```python
from build123d import *

# Parameters (mm, degrees)
CROQUIS1_R              = 13
CROQUIS1_R_2            = 5
SALIENTE_EXTRUIR1_DEPTH = 8
CHAFL_N1_SIZE           = 0.3
CROQUIS2_W              = 1
CROQUIS2_H              = 0.2


with BuildPart() as part:
    # Croquis1 → Saliente-Extruir1 (new body)
    with BuildSketch(Plane.XY):
        Circle(CROQUIS1_R)
        Circle(CROQUIS1_R_2, mode=Mode.SUBTRACT)
    extrude(amount=SALIENTE_EXTRUIR1_DEPTH)

    # Chaflán1
    chafl_n1_edges = [part.edges().sort_by_distance(p)[0] for p in [
        (-13, 0, 0),
        (-13, 0, 8),
        (-5, 0, 0),
        (-5, 0, 8),
    ]]
    chamfer(chafl_n1_edges, length=CHAFL_N1_SIZE)

    # Croquis2 → Cortar-Revolución1 (revolve, cut)
    with BuildSketch(Plane(origin=(0, 0, 0), x_dir=(0, 0, -1), z_dir=(1, 0, 0))):
        Polygon((-8.85, 11.267505128), (-7.85, 11.142505128), (-7.85, 10.892505128), (-8.85, 10.767505128), align=None)
        Polygon((0.85, 10.767505128), (0.85, 11.267505128), (-0.15, 11.142505128), (-0.15, 10.892505128), align=None)
        with Locations((-8.35, 7.665073065)):
            Rectangle(CROQUIS2_W, CROQUIS2_H)
        with Locations((0.35, 7.665073065)):
            Rectangle(CROQUIS2_W, CROQUIS2_H)
    revolve(axis=Axis((0, 0, 12.411349243), (0, 0, -1)), mode=Mode.SUBTRACT)


solid = part.part
```
Geometry: final body of the model. Coordinates: model frame, mm. Give positions to 0.01 mm unless a question says otherwise; leave off trailing zeros. Order: outer loops, then holes, each group sorted by start corner. A loop starts at its lowest first (then second) coordinate and runs counter-clockwise, first axis right, second up. Notation, with made-up numbers: M 22.25,-7.75 L 57.25,-7.75 A13 cw 57.25,13.25 Z; hole C -15,-4 d9. An arc over 180 degrees is marked long. Answer as CSV lines item,"result". Start each with the question number.
1) Mould query, pull axis Y, two halves, no side actions, for faces 1 (the cylindrical face through (-10.316, -7.91, 3.948)), 2 (the flat face through (5, -7, 8)), 3 (the cylindrical face through (-1.08, -4.88, 3.95)). Classes: +Y half, -Y half, draft (parallel to the pull), parting line (faces both ways), or undercut.
2) Cut plane A-A (z = 3.75). Output: boundary loops of the cut face in (x, y).
3) Line query: line 1 (X direction, y = 0.25, z = 1.25); line 2 (Z direction, x = -10.75, y = -2.5); line 3 (X direction, y = 1, z = 5.5). Output: solid intervals per line, ascending. Write a range as from..to.
4) First-contact query: P1, Ø4.5, axis at x = -3.5, y = -3.5, coming from the -Z side; P2, Ø6, axis at x = 0, y = 0, coming from the -Z side; P3, Ø4, axis at x = 4.5, z = 2, coming from the -Y side. Flat tips, straight axial feed; report the tip coordinate or a pass-through.
Findings below:
1,face 1,"parting line"
1,face 2,"draft"
1,face 3,"undercut"
2,outline,"C 0,0 d26; hole C 0,0 d10"
3,line 1,"x = -13..-4.99, 4.99..13"
3,line 2,"z = 0.15..7.85"
3,line 3,"x = -12.96..-4.9, 4.9..12.96"
4,P1,"stops at z = 0"
4,P2,"passes through"
4,P3,"stops at y = -12.76"
